The listing builds one solid part. Answer for the finished solid, in the listing's coordinates (mm). Face numbers are marked on the shaded views. A direction names the side the tool comes from. Give positions to 0.01 mm unless a question says otherwise; leave off trailing zeros. Write each loop counter-clockwise with the first axis right and the second up, starting at its lowest first coordinate (ties: lowest second). Pieces come first, ordered by that corner, then holes. Notation, with made-up numbers: (47, -38.5) - (83, -38.5) arc R17 ccw to (83, -15.5) - close; hole circle Ø8 at (74.5, 37.25). An arc over 180 degrees is marked (long way). Return JSON: item names as keys, results as strings.
from build123d import *

# Parameters (mm, degrees)
F0_W            = 77
F0_H            = 144
F1_DEPTH        = 13
F3_DEPTH        = 142
F4_W            = 65
F4_H            = 2
F5_DEPTH        = 4
F6_W            = 10.5
F6_H            = 7.5
F7_DEPTH        = 25
F8_W            = 8.0420786627
F8_H            = 42
F9_DEPTH        = 25
F10_W           = 77
F10_H           = 54
F10_W_2         = 36
F11_DEPTH       = 50
F13_DEPTH       = 111
F14_W           = 38
F14_H           = 2
F15_DEPTH       = 4
F16_DEPTH       = 8
F17_W           = 50
F17_H           = 25.4
F18_DEPTH       = 5
F20_D           = 6.35
F20_DEPTH       = 8
F20_CBORE_D     = 14
F20_CBORE_DEPTH = 3.175
F20_TIP         = 1.9077324654
F21_R           = 5


with BuildPart() as f1:
    # F0 (on Front) → F1 (new body)
    with BuildSketch(Plane.XZ):
        Rectangle(F0_W, F0_H)
    extrude(amount=F1_DEPTH)

    # F2 (on face) → F3 (cut)
    with BuildSketch(Plane.XY.offset(72)):
        Polygon((-32.5, -11), (-32.5, -13), (32.5, -13), (32.5, -11), (36.5, -11), (36.5, -2), (-36.5, -2), (-36.5, -11), align=None)
    extrude(amount=-F3_DEPTH, mode=Mode.SUBTRACT)

    # F4 (on face) → F5 (join)
    with BuildSketch(Plane.XY.offset(-70)):
        with Locations((0, -12)):
            Rectangle(F4_W, F4_H)
    extrude(amount=F5_DEPTH)

    # F6 (on face) → F7 (cut)
    with BuildSketch(Plane(origin=(0, 0, -72), x_dir=(1, 0, 0), z_dir=(0, 0, -1))):
        with Locations((0, 6.5)):
            Rectangle(F6_W, F6_H)
    extrude(amount=-F7_DEPTH, mode=Mode.SUBTRACT)

    # F8 (on face) → F9 (cut)
    with BuildSketch(Plane.YZ.offset(38.5)):
        with Locations((-6.5, 20)):
            Rectangle(F8_W, F8_H)
    extrude(amount=-F9_DEPTH, mode=Mode.SUBTRACT)

    # F10 (on face) → F11 (join)
    with BuildSketch(Plane(origin=(0, 0, 0), x_dir=(-1, 0, 0), z_dir=(0, 1, 0))):
        with Locations((0, 25)):
            Rectangle(F10_W, F10_H)
        with Locations((-56.5, 25)):
            Rectangle(F10_W_2, F10_H)
    extrude(amount=F11_DEPTH)

    # F12 (on face) → F13 (cut)
    with BuildSketch(Plane(origin=(-38.5, 0, 0), x_dir=(0, -1, 0), z_dir=(-1, 0, 0))):
        Polygon((-6, 50), (-6, 52), (-44, 52), (-44, 50), (-48, 50), (-48, 2), (-2, 2), (-2, 50), align=None)
    extrude(amount=-F13_DEPTH, mode=Mode.SUBTRACT)

    # F14 (on face) → F15 (join)
    with BuildSketch(Plane(origin=(72.5, 0, 0), x_dir=(0, -1, 0), z_dir=(-1, 0, 0))):
        with Locations((-25, 51)):
            Rectangle(F14_W, F14_H)
    extrude(amount=F15_DEPTH)

    # F16 (add): a face of the model
    f16_faces = [f1.faces().sort_by_distance(p)[0] for p in [
        (18, 25, -2),
    ]]
    extrude(f16_faces, amount=F16_DEPTH)

    # F17 (on face) → F18 (cut)
    with BuildSketch(Plane(origin=(0, 0, -10), x_dir=(1, 0, 0), z_dir=(0, 0, -1))):
        with Locations((49.5, -20.2)):
            Rectangle(F17_W, F17_H)
    extrude(amount=-F18_DEPTH, mode=Mode.SUBTRACT)

    # F20
    with Locations(Plane.XY.offset(2)):
        with Locations((62.5, 20.2), (37.5, 20.2)):
            CounterBoreHole(F20_D / 2, F20_CBORE_D / 2, F20_CBORE_DEPTH, depth=F20_DEPTH)
            with Locations((0, 0, -(F20_DEPTH + F20_TIP / 2))):  # 118° drill point
                Cone(0, F20_D / 2, F20_TIP, mode=Mode.SUBTRACT)

    # F21
    f21_edges = [f1.edges().sort_by_distance(p)[0] for p in [
        (0, 0, -10),
        (0, 0, 52),
    ]]
    fillet(f21_edges, radius=F21_R)


solid = f1.part
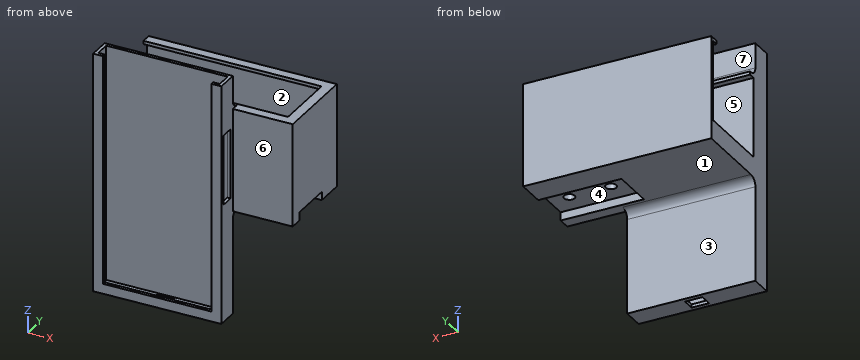
Item 1: The mould has two halves that part along Y. Classify the marked faces 1, 2 and 3: +Y half, -Y half, draft (parallel to the pull), parting line (faces both ways), or undercut.
Answer below:
{"face 1": "draft", "face 2": "undercut", "face 3": "+Y half"}
Item 2: For the marked faces 4, 5, 6 and 7, determine the directions among +Z, -Z, +X, -X, +Y, -Y from which every point of the face is accessible in a straight line to the end or side of a thin tool.
Answer below:
{"face 4": "-Z, +X", "face 5": "-X", "face 6": "+Z, -Z, +X, -Y", "face 7": "+Z, +X, -X, +Y"}
Item 3: A cutting plane is placed at D-D on x = 62.5. Determine the outline of the cut face in (y, z) (3 decimals).
Answer below:
{"outline": "(0, -10) - (7.5, -10) - (7.5, -5) - (17.025, -5) - (17.025, -1.175) - (13.2, -1.175) - (13.2, 2) - (2, 2) - (2, 50) - (6, 50) - (6, 52) - (0, 52) - close; (23.375, -5) - (32.9, -5) - (32.9, -10) - (50, -10) - (50, 52) - (44, 52) - (44, 50) - (48, 50) - (48, 2) - (27.2, 2) - (27.2, -1.175) - (23.375, -1.175) - close"}
Item 4: Flat-ended cylindrical pins translate along their axes: P1, Ø12, axis at x = 11.5, z = 64.5, coming from the +Y side; P2, Ø5.5, axis at y = -5, z = 20.5, coming from the +X side; P3, Ø1.5, axis at x = -14, y = 38.5, coming from the +Z side. Find the tip coordinate at first contact, or state that the pin passes through.
Answer below:
{"P1": "stops at y = 0", "P2": "stops at x = 38.5", "P3": "stops at z = 2"}
Item 5: A cutting plane is placed at A-A on y = -5. Determine the outline of the cut face in (x, z).
Answer below:
{"outline": "(-38.5, -72) - (-5.25, -72) - (-5.25, -70) - (-36.5, -70) - (-36.5, 72) - (-38.5, 72) - close; (5.25, -72) - (38.5, -72) - (38.5, -1) - (36.5, -1) - (36.5, -70) - (5.25, -70) - close; (36.5, 41) - (38.5, 41) - (38.5, 72) - (36.5, 72) - close"}
Item 6: A cutting plane is placed at C-C on y = 42. Determine the outline of the cut face in (x, z).
Answer below:
{"outline": "(-38.5, -10) - (74.5, -10) - (74.5, 52) - (68.5, 52) - (68.5, 50) - (72.5, 50) - (72.5, 2) - (-38.5, 2) - close"}
Item 7: Consider L1, parallel to Y at x = 37.5, z = 0.55; L2, parallel to X at y = 20, z = -2; L3, parallel to Y at x = 62.5, z = -3.75 (3 decimals). Determine where each line is inside the solid, lowest interval first.
Answer below:
{"L1": "y = -13 to -10.52, -2.48 to 13.2, 27.2 to 50", "L2": "x = -38.5 to 34.33, 40.67 to 59.33, 65.67 to 74.5", "L3": "y = 0 to 17.025, 23.375 to 50"}
Item 8: A cutting plane is placed at B-B on x = -1. Determine the outline of the cut face in (y, z).
Answer below:
{"outline": "(-13, -72) - (-10.25, -72) - (-10.25, -70) - (-11, -70) - (-11, -66) - (-13, -66) - close; (-2.75, -72) - (0, -72) - (0, -15) arc R5 cw to (5, -10) - (50, -10) - (50, 52) - (44, 52) - (44, 50) - (48, 50) - (48, 2) - (2, 2) - (2, 50) - (6, 50) - (6, 52) - (5, 52) arc R5 cw to (0, 57) - (0, 72) - (-2, 72) - (-2, -70) - (-2.75, -70) - close"}
